Geometry check sheet. Reference: the model listing, model coordinates, mm. A direction names the side the tool comes from. Give positions to 0.01 mm unless a question says otherwise; leave off trailing zeros. Loops run counter-clockwise (first coordinate to the right, second up) from the corner with the lowest first, then second, coordinate; pieces in that order, holes last. Notation, with made-up numbers: (-33, -15) - (-18, -15) arc R24 cw to (-18, 9) - close; hole circle Ø1 at (10, 44). An arc over 180 degrees is marked (long way). Use a Markdown table: item, result. Add a question column.
1. Set-up check for faces 1 (the flat face through (-8, -30, 13)), 2 (the flat face through (16, 1, 40)): record each of +Z, -Z, +X, -X, +Y, -Y from which the full face is reachable in a straight line by a thin tool's end or side.
2. Cross-section at B-B on z = 16.5. Enter the section's corners in (x, y), and give its area (3 significant figures).
3. Cross-section at D-D on z = 28.5. Enter the section's corners in (x, y).
4. Material ranges on L1, parallel to Y at x = 0, z = 20.5; L2, parallel to Z at x = -33.5, y = 15; L3, parallel to Y at x = 14.5, z = 31, recorded low to high.
5. Depth check by flat-ended pin: P1, Ø5, axis at y = 25.5, z = 31, coming from the -X side; P2, Ø3, axis at y = 24, z = 20, coming from the -X side; P3, Ø6, axis at x = -3, y = -25, coming from the +Z side. Enter the tip coordinate at first touch or a pass-through.
6. Draft check along Y on faces 3 (the flat face through (0, 0, 39)), 4 (the cylindrical face through (11.923, 3.755, 40.493)), 5 (the conical face through (12.77, 4.02, 38.11)), 6 (the flat face through (0, 0, 41)). Enter one of: pulls with the +Y half, pulls with the -Y half, needs draft (parallel to the pull), parting line crosses it, or undercut.
7. Cross-section at A-A on x = 0. Enter the section's corners in (y, z), and give its area (3 significant figures).
from build123d import *

# Parameters (mm, degrees)
F0_R        = 36.75
F0_R_2      = 30.75
F1_DEPTH    = 40
F2_START    = 20
F0_R_3      = 12.5
F2_DEPTH    = 20
F3_START    = 39
F3_DEPTH    = 2
F4_S5_R     = 30.75
F4_T6_DEPTH = 47
F5_DEPTH    = 13


# Not quite as in the source:
# - a fillet or chamfer that OpenCascade refuses, or shapes differently, is made with other operations: its cross-section is extruded or revolved along the edge and cut away or added


with BuildPart() as f1:
    # F0 (on Top) → F1 (new body)
    with BuildSketch(Plane.XY):
        Circle(F0_R)
        Circle(F0_R_2, mode=Mode.SUBTRACT)
    extrude(amount=F1_DEPTH)

    # F0 (on Top) → F2 (join)
    with BuildSketch(Plane.XY.offset(F2_START)):
        Circle(F0_R_2)
        Circle(F0_R_3, mode=Mode.SUBTRACT)
    extrude(amount=F2_DEPTH)

    # F0 (on Top) → F3 (join)
    with BuildSketch(Plane.XY.offset(F3_START)):
        Circle(F0_R_3)
    extrude(amount=F3_DEPTH)

    # F4: chamfer of 19 on 1 edges, made by hand


with BuildPart() as f4_tool2:
    # F4_s3 → F4_t4 (revolve)
    with BuildSketch(Plane.XZ):
        Polygon((31.5, 20), (12.5, 39), (12.5, 20), align=None)
    revolve(axis=Axis((0, 0, 20), (0, 0, 1)))

    # F4_s5 → F4_t6 (intersect, symmetric)
    with BuildSketch(Plane.XY.offset(29.5)):
        Circle(F4_S5_R)
    extrude(amount=F4_T6_DEPTH, both=True, mode=Mode.INTERSECT)

    split(bisect_by=Plane.XY.offset(39), keep=Keep.BOTTOM)


with BuildPart() as f1_1:
    add(f1.part)

    # F4_t1: cut F4_tool2
    add(f4_tool2.part, mode=Mode.SUBTRACT)

    # F5 (cut): a face of the model
    f5_faces = [f1_1.faces().sort_by_distance(p)[0] for p in [
        (-35.7105530317, 0, 0),
    ]]
    extrude(f5_faces, amount=-F5_DEPTH, mode=Mode.SUBTRACT)


solid = f1_1.part
Values found:
| question | item | result |
|---|---|---|
| 1 | face 1 | -Z, +X, -X, +Y, -Y |
| 1 | face 2 | +Z |
| 2 | outline | circle Ø73.5 at (0, 0); hole circle Ø61.5 at (0, 0) |
| 2 | area | 1,270 mm2 |
| 3 | outline | circle Ø73.5 at (0, 0); hole circle Ø46 at (0, 0) |
| 4 | L1 | y = -36.75 to -30.75, 30.75 to 36.75 |
| 4 | L2 | z = 13 to 40 |
| 4 | L3 | y = -33.77 to -14.49, 14.49 to 33.77 |
| 5 | P1 | stops at x = -28.66 |
| 5 | P2 | stops at x = -29.06 |
| 5 | P3 | stops at z = 40 |
| 6 | face 3 | undercut |
| 6 | face 4 | parting line crosses it |
| 6 | face 5 | undercut |
| 6 | face 6 | needs draft |
| 7 | outline | (-36.75, 13) - (-30.75, 13) - (-30.75, 20.75) - (-12.5, 39) - (12.5, 39) - (30.75, 20.75) - (30.75, 13) - (36.75, 13) - (36.75, 40) - (12.5, 40) - (12.5, 41) - (-12.5, 41) - (-12.5, 40) - (-36.75, 40) - close |
| 7 | area | 744 mm2 |
